Check sheet for the modelled part. Datum: model origin and axes. Units: mm. Round coordinates to 2 decimals unless told otherwise and drop trailing zeros. Order: outer loops, then holes, each group sorted by start corner. A loop starts at its lowest first (then second) coordinate and runs counter-clockwise, first axis right, second up.
Q1. Cross-section at B-B on z = 0.45. Record the cut outline in (x, y), then the cut area to 3 significant figures.
Q2. Cross-section at A-A on y = -7.5. Record the cut outline in (x, z).
Q3. Scan lines: probe 1 along Y at (x, z) = (-5, 1.2); probe 2 along X at (y, z) = (-11, 1.95); probe 3 along X at (y, z) = (8.75, 0.25). Record each from-to range of solid material in increasing order.
Q4. Cross-section at C-C on x = -10. Record the cut outline in (y, z).
from build123d import *

# Parameters (mm, degrees)
SKETCH_1_W      = 29
SKETCH_1_H      = 21
SKETCH_1_R      = 1.6
SKETCH_1_W_2    = 8
SKETCH_1_H_2    = 2.1
EXTRUDE_1_DEPTH = 2


with BuildPart() as part:
    # 草图1 → 凸台-拉伸1 (new body)
    # profile 1 of 5: a face of its own
    with BuildSketch(Plane.XY):
        with Locations((-10.082297853, 0)):
            Rectangle(SKETCH_1_W, SKETCH_1_H)
        with Locations((-15.082297853, 7.5)):
            Circle(SKETCH_1_R, mode=Mode.SUBTRACT)
        with Locations((-5.082297853, 7.5)):
            Circle(SKETCH_1_R, mode=Mode.SUBTRACT)
        with Locations((-15.082297853, -7.5)):
            Circle(SKETCH_1_R, mode=Mode.SUBTRACT)
        with Locations((-5.082297853, -7.5)):
            Circle(SKETCH_1_R, mode=Mode.SUBTRACT)
    # profile 2 of 5: a face of its own
    with BuildSketch(Plane.XY):
        with Locations((-20.582297853, 11.55)):
            Rectangle(SKETCH_1_W_2, SKETCH_1_H_2)
    # profile 3 of 5: a face of its own
    with BuildSketch(Plane.XY):
        with Locations((0.417702147, 11.55)):
            Rectangle(SKETCH_1_W_2, SKETCH_1_H_2)
    # profile 4 of 5: a face of its own
    with BuildSketch(Plane.XY):
        with Locations((-20.582297853, -11.55)):
            Rectangle(SKETCH_1_W_2, SKETCH_1_H_2)
    # profile 5 of 5: a face of its own
    with BuildSketch(Plane.XY):
        with Locations((0.417702147, -11.55)):
            Rectangle(SKETCH_1_W_2, SKETCH_1_H_2)
    extrude(amount=EXTRUDE_1_DEPTH)


solid = part.part
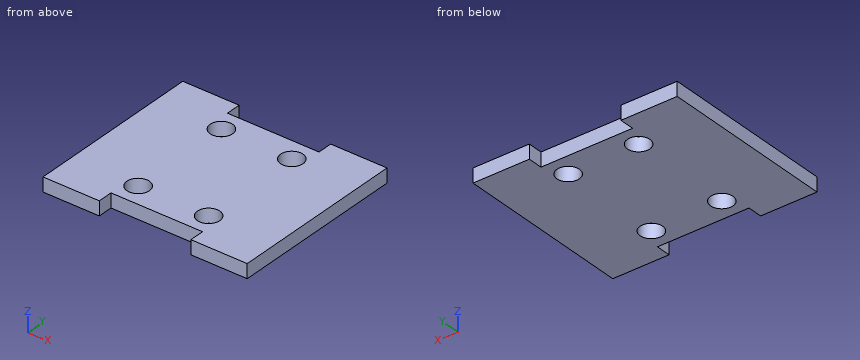
Results found:
1. outline: (-24.58, -12.6) - (-16.58, -12.6) - (-16.58, -10.5) - (-3.58, -10.5) - (-3.58, -12.6) - (4.42, -12.6) - (4.42, 12.6) - (-3.58, 12.6) - (-3.58, 10.5) - (-16.58, 10.5) - (-16.58, 12.6) - (-24.58, 12.6) - close; hole circle Ø3.2 at (-15.08, -7.5); hole circle Ø3.2 at (-15.08, 7.5); hole circle Ø3.2 at (-5.08, -7.5); hole circle Ø3.2 at (-5.08, 7.5)
1. area: 644 mm2
2. outline: (-24.58, 0) - (-16.68, 0) - (-16.68, 2) - (-24.58, 2) - close; (-13.48, 0) - (-6.68, 0) - (-6.68, 2) - (-13.48, 2) - close; (-3.48, 0) - (4.42, 0) - (4.42, 2) - (-3.48, 2) - close
3. probe 1: y = -10.5 to -9.1, -5.9 to 5.9, 9.1 to 10.5
3. probe 2: x = -24.58 to -16.58, -3.58 to 4.42
3. probe 3: x = -24.58 to -16.08, -14.08 to -6.08, -4.08 to 4.42
4. outline: (-10.5, 0) - (10.5, 0) - (10.5, 2) - (-10.5, 2) - close
